```python
from build123d import *

# Parameters (mm, degrees)
SKETCH1_W           = 635
SKETCH1_H           = 101.6
BOSS_EXTRUDE1_DEPTH = 35.052
CUT_EXTRUDE3_START  = -1
SKETCH1_3_R         = 15.08125
CUT_EXTRUDE3_DEPTH  = 37.052
LPATTERN1_COUNT     = 18
LPATTERN1_PITCH     = 33.9725


with BuildPart() as part:
    # Sketch1 → Boss-Extrude1 (new body)
    with BuildSketch(Plane(origin=(0, 0, 0), x_dir=(1, 0, 0), z_dir=(0, 1, 0))):
        with Locations((-279.0825, 0)):
            Rectangle(SKETCH1_W, SKETCH1_H)
    extrude(amount=BOSS_EXTRUDE1_DEPTH)

    # Sketch1<3> → Cut-Extrude3 (cut)
    with BuildSketch(Plane(origin=(0, 0, 0), x_dir=(1, 0, 0), z_dir=(0, 1, 0)).offset(CUT_EXTRUDE3_START)):
        Circle(SKETCH1_3_R)
        with Locations((16.98625, 29.21)):
            Circle(SKETCH1_3_R)
        with Locations((16.98625, -29.21)):
            Circle(SKETCH1_3_R)
    cut_extrude3 = extrude(amount=CUT_EXTRUDE3_DEPTH, mode=Mode.SUBTRACT)

    # LPattern1: Cut-Extrude3 ×18
    with Locations(*[(-i * LPATTERN1_PITCH, 0, 0) for i in range(1, LPATTERN1_COUNT)]):
        add(cut_extrude3, mode=Mode.SUBTRACT)


solid = part.part
```
Model file for the job. Use its own axes, mm. Give positions to 0.01 mm unless a question says otherwise; leave off trailing zeros. Order: outer loops, then holes, each group sorted by start corner. A loop starts at its lowest first (then second) coordinate and runs counter-clockwise, first axis right, second up.
1) Saw through at A-A, the plane x = -553. Write the cut outline in (y, z).
2) Wall check: probe 1 along Z at (x, y) = (-322, 14); probe 2 along Z at (x, y) = (-373.5, 12); probe 3 along Z at (x, y) = (-275, 16). Give the ranges that are in metal, low to high.
3) Saw through at B-B, the plane z = -29.21. Count the separate pieces of the cut face and the enclosed holes in it, then the cut area to 3 significant figures.
Computed:
1. outline: (0, -50.8) - (35.05, -50.8) - (35.05, -42.27) - (0, -42.27) - close; (0, -16.15) - (35.05, -16.15) - (35.05, -11.76) - (0, -11.76) - close; (0, 11.76) - (35.05, 11.76) - (35.05, 16.15) - (0, 16.15) - close; (0, 42.27) - (35.05, 42.27) - (35.05, 50.8) - (0, 50.8) - close
2. probe 1: z = -50.8 to -44.27, -14.15 to 14.15, 44.27 to 50.8
2. probe 2: z = -50.8 to -15.08, 15.08 to 50.8
2. probe 3: z = -50.8 to -35.37, -23.05 to -14.73, 14.73 to 23.05, 35.37 to 50.8
3. separate pieces: 19
3. enclosed holes: 0
3. area: 3,230 mm2
